Source: CAD feature listing. Evaluate the final solid. Frame: model axes, mm. A direction names the side the tool comes from. Coordinates: 2 decimals unless noted, no trailing zeros. Loops run counter-clockwise (first coordinate to the right, second up) from the corner with the lowest first, then second, coordinate; pieces in that order, holes last. Notation, with made-up numbers: (-22, 80) -> (-1, 80) arc R8 ccw to (-1, 94) -> close; hole circle Ø7 at (12, 15.5). An arc over 180 degrees is marked (long way). Answer as a JSON object with one key per item and string values. Group by question number.
from build123d import *

# Parameters (mm, degrees)
F0_R     = 1.8
F1_DEPTH = 6


# Not quite as in the source:
# - a feature names something its author has since deleted; it is built from what else it names


with BuildPart() as f1:
    # F0 (on Top) → F1 (new body)
    with BuildSketch(Plane.XY):
        with BuildLine():
            ThreePointArc((-26.9197331922, -29.0044), (-22.202470707, -26.7069691338), (-18.925, -30.8044))
            ThreePointArc((-18.925, -30.8044), (-22.202470707, -34.9018308662), (-26.9197331922, -32.6044))
            Line((-26.9197331922, -32.6044), (-30.2622788846, -32.6044))
            Line((-30.2622788846, -32.6044), (-30.2622788846, -33.8044))
            Line((-30.2622788846, -33.8044), (-33.2622788846, -33.8044))
            Line((-33.2622788846, -33.8044), (-33.2622788846, -32.6044))
            Line((-33.2622788846, -32.6044), (-35.8254, -32.6044))
            Line((-35.8254, -32.6044), (-35.8254, -35.0044))
            ThreePointArc((-35.8254, -35.0044), (-34.3609339059, -38.5399339059), (-30.8254, -40.0044))
            Line((-30.8254, -40.0044), (-19.625, -40.0044))
            ThreePointArc((-19.625, -40.0044), (-16.0894660941, -38.5399339059), (-14.625, -35.0044))
            Line((-14.625, -35.0044), (-14.625, -25.0977827265))
            ThreePointArc((-14.625, -25.0977827265), (-14.400006794, -23.6147756066), (-13.7452759529, -22.2652350973))
            Line((-13.7452759529, -22.2652350973), (-11.8023123147, -19.4389644026))
            Line((-11.8023123147, -19.4389644026), (4.5746, 2.4))
            Line((4.5746, 2.4), (36.6099, 2.4))
            Line((36.6099, 2.4), (36.6099, 11.6009423509))
            Line((36.6099, 11.6009423509), (37.1099, 11.6009423509))
            Line((37.1099, 11.6009423509), (38.9099, 11.6009423509))
            Line((38.9099, 11.6009423509), (40.7099, 11.6009423509))
            Line((40.7099, 11.6009423509), (41.2099, 11.6009423509))
            Line((41.2099, 11.6009423509), (41.2099, 1.8140082314))
            Line((41.2099, 1.8140082314), (48.4484305441, 1.8140082314))
            Line((48.4484305441, 1.8140082314), (48.4484305441, 15.1736566274))
            ThreePointArc((48.4484305441, 15.1736566274), (48.3232531582, 16.2854589848), (47.9539887514, 17.341592337))
            Line((47.9539887514, 17.341592337), (41.9726020282, 29.7725357096))
            ThreePointArc((41.9726020282, 29.7725357096), (40.1857248711, 31.8008808947), (37.6042192016, 32.6027179373))
            ThreePointArc((37.6042192016, 32.6027179373), (37.1447174672, 32.5688699786), (36.6902824172, 32.4928679158))
            Line((36.6902824172, 32.4928679158), (-31.8765121651, 17.7491195886))
            ThreePointArc((-31.8765121651, 17.7491195886), (-34.7148447435, 16.0028605187), (-35.8254, 12.8608516729))
            Line((-35.8254, 12.8608516729), (-35.8254, 2.4))
            Line((-35.8254, 2.4), (-25.4254, 2.4))
            Line((-25.4254, 2.4), (-25.4254, 1.9))
            Line((-25.4254, 1.9), (-25.4254, -1.7))
            Line((-25.4254, -1.7), (-25.4254, -2.2))
            Line((-25.4254, -2.2), (-35.8254, -2.2))
            Line((-35.8254, -2.2), (-35.8254, -29.0044))
            Line((-35.8254, -29.0044), (-33.2622788846, -29.0044))
            Line((-33.2622788846, -29.0044), (-33.2622788846, -27.8044))
            Line((-33.2622788846, -27.8044), (-30.2622788846, -27.8044))
            Line((-30.2622788846, -27.8044), (-30.2622788846, -29.0044))
            Line((-30.2622788846, -29.0044), (-26.9197331922, -29.0044))
        make_face()
        with Locations((-5.5901, 0.1)):
            Circle(F0_R, mode=Mode.SUBTRACT)
        with Locations((38.9099, 22.2547)):
            Circle(F0_R, mode=Mode.SUBTRACT)
    extrude(amount=F1_DEPTH)


solid = f1.part
1. Section query D-D on x = 15.5. Return loops of the section in (y, z), then the cut area to 3 significant figures.
2. Section query B-B on z = 4.4. State how many separate pieces and enclosed holes the cut face has, then the cut area to 3 significant figures.
3. Pin query (flat end, axial travel): pin 1 Ø1.3 at (x, z) = (-34.5, 2.5) entering from -Y; pin 2 Ø1.8 at (x, z) = (-32.5, 3.5) entering from -Y; pin 3 Ø1.5 at (x, z) = (17, 2) entering from +Y; pin 4 Ø6 at (x, y) = (-19.5, 12.5) entering from -Z. Return the tip coordinate at first contact, or that it passes through.
4. Section query C-C on y = -16.5. Return loops of the section in (x, z).
5. Ray query, L1, parallel to X at y = 11, z = 5.4; L2, parallel to X at y = 0, z = 2.25; L3, parallel to Y at x = -27, z = 4.1. Return the intervals inside material, ascending.
6. Section query A-A on y = 0.1. Return loops of the section in (x, z), then the cut area to 3 significant figures.
7. Reachability of faces 1 (the face through (45.005, 23.47, 2.958)), 2 (the face through (-14.625, -30, 3)), 3 (the face through (-35, -32.604, 3)) from +Z, -Z, +X, -X, +Y, -Y: full face, straight path, thin tool, end or side. Return the list, or none.
8. Mould query, pull axis X, two halves, no side actions, for faces 4 (the face through (41.21, 7, 3)), 5 (the face through (36.61, 7, 3)), 6 (the face through (2.887, 25.224, 2.958)), 7 (the face through (-14.406, -23.635, 2.958)). Classes: pulls with the +X half, pulls with the -X half, needs draft (parallel to the pull), parting line crosses it, or undercut.
Solved:
{
 "1": {"outline": "(2.4, 0) -> (27.94, 0) -> (27.94, 6) -> (2.4, 6) -> close", "area": "153 mm^2"},
 "2": {"separate pieces": "1", "enclosed holes": "2", "area": "2,840 mm^2"},
 "3": {"pin 1": "y = -38.99", "pin 2": "y = -39.94", "pin 3": "y = 28.42", "pin 4": "z = 0"},
 "4": {"outline": "(-35.83, 0) -> (-9.6, 0) -> (-9.6, 6) -> (-35.83, 6) -> close"},
 "5": {"L1": "-35.83 to 36.61, 41.21 to 48.45", "L2": "-25.43 to -7.39, -3.79 to 2.77", "L3": "-40 to -32.6, -29 to -2.2, 2.4 to 18.8"},
 "6": {"outline": "(-25.43, 0) -> (-7.39, 0) -> (-7.39, 6) -> (-25.43, 6) -> close; (-3.79, 0) -> (2.85, 0) -> (2.85, 6) -> (-3.79, 6) -> close", "area": "148 mm^2"},
 "7": {"face 1": "+Z, -Z, +X, +Y", "face 2": "+Z, -Z, +X, -Y", "face 3": "+Z, -Z, -X"},
 "8": {"face 4": "undercut", "face 5": "undercut", "face 6": "pulls with the -X half", "face 7": "pulls with the +X half"}
}
